Part print with two shaded views. Sizes in mm from the minimum x, y, z corner. A direction names the side the tool comes from. Give positions to 0.01 mm unless a question says otherwise; leave off trailing zeros. Write each loop counter-clockwise with the first axis right and the second up, starting at its lowest first coordinate (ties: lowest second). Pieces come first, ordered by that corner, then holes. Notation, with made-up numbers: (35, 5.5) -> (65, 5.5) arc R24 cw to (65, 44.5) -> close; hole circle Ø4 at (50, 71.5). An arc over 180 degrees is marked (long way). Answer in a Markdown table with one row per item. Add a question column.
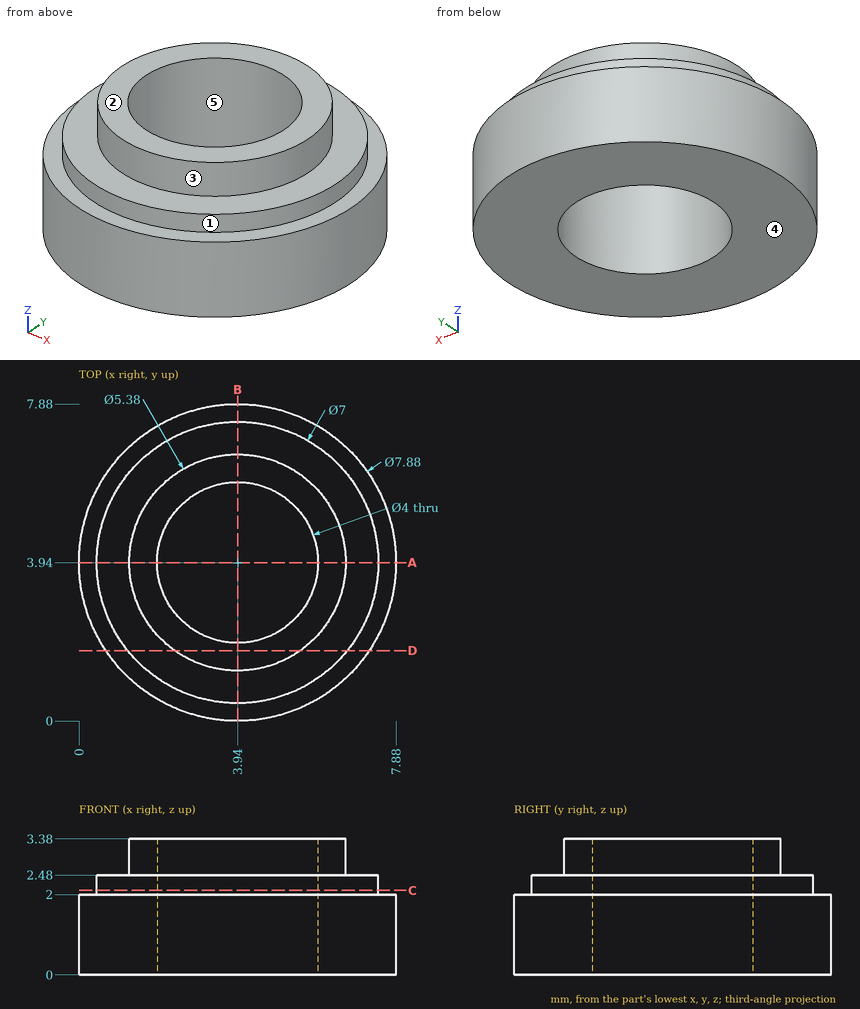
Item 1: Slice it at D-D, the plane y = 1.75. List the corners of the cut face in (x, z).
Item 2: Drop a flat-ended pin along its axis: pin 1 Ø2.5 at (x, y) = (4.5, 3.5) entering from +Z. Give the stop position or say it passes through.
Item 3: Which spindle directions (+Z, -Z, +X, -X, +Y, -Y) get a long thin tool onto all of the face, cutting with end or side? Do the marked faces 1 and 2. Say none if no direction does.
Item 4: Mould opens along Y. For the marked faces 3, 4 and 5 say: released by +Y, released by -Y, zero draft, split by the parting line, or undercut.
Item 5: Slice it at C-C, the plane z = 2.1. List the corners of the cut face in (x, y).
Item 6: Slice it at A-A, the plane y = 3.94. List the corners of the cut face in (x, z), then the cut area to 3 significant figures.
Item 7: Probe L1, parallel to Y at x = 3.94, z = 0.8; L2, parallel to X at y = 3.94, z = 2.1; L3, parallel to Z at x = 4, y = 0.5. List the from-to ranges inside material, lowest first. Write a range as from..to.
Answer key:
| question | item | result |
|---|---|---|
| 1 | outline | (0.66, 0) -> (7.22, 0) -> (7.22, 2) -> (6.67, 2) -> (6.67, 2.48) -> (5.5, 2.48) -> (5.5, 3.38) -> (2.38, 3.38) -> (2.38, 2.48) -> (1.21, 2.48) -> (1.21, 2) -> (0.66, 2) -> close |
| 2 | pin 1 | passes through |
| 3 | face 1 | +Z |
| 3 | face 2 | +Z, +X, -X, +Y, -Y |
| 4 | face 3 | split by the parting line |
| 4 | face 4 | zero draft |
| 4 | face 5 | undercut |
| 5 | outline | circle Ø7 at (3.94, 3.94); hole circle Ø4 at (3.94, 3.94) |
| 6 | outline | (0, 0) -> (1.94, 0) -> (1.94, 3.38) -> (1.25, 3.38) -> (1.25, 2.48) -> (0.44, 2.48) -> (0.44, 2) -> (0, 2) -> close; (5.94, 0) -> (7.88, 0) -> (7.88, 2) -> (7.44, 2) -> (7.44, 2.48) -> (6.63, 2.48) -> (6.63, 3.38) -> (5.94, 3.38) -> close |
| 6 | area | 10.4 mm² |
| 7 | L1 | y = 0..1.94, 5.94..7.88 |
| 7 | L2 | x = 0.44..1.94, 5.94..7.44 |
| 7 | L3 | z = 0..2.48 |
